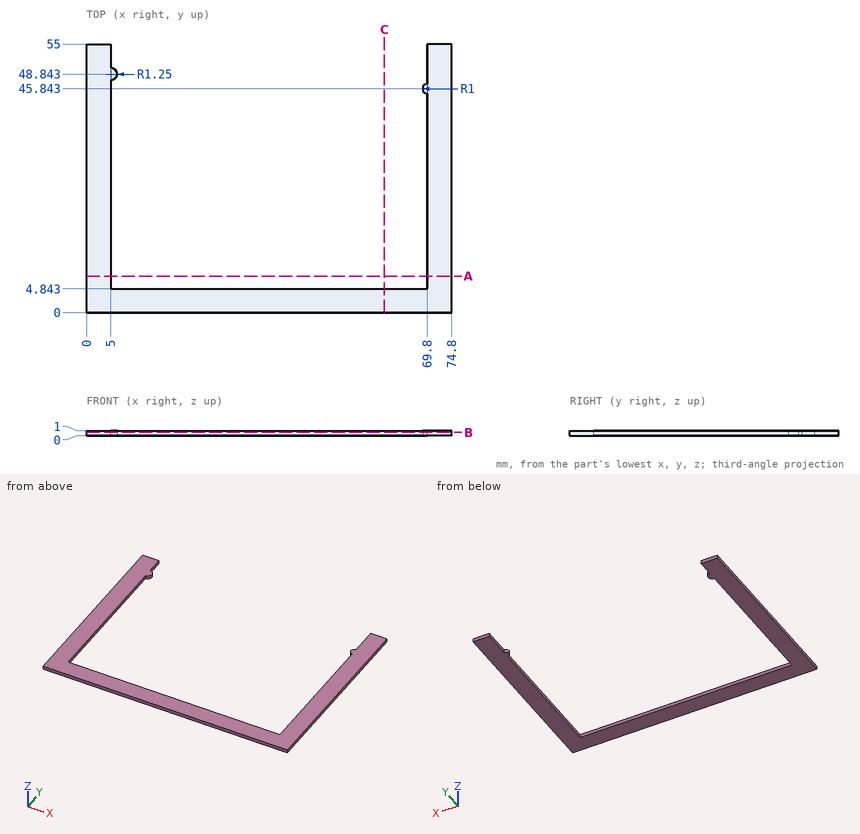
Here's the drawing with two shaded views (mm, measured from the low corner). I have some questions. Coordinates: 2 decimals unless noted, no trailing zeros. Write each loop counter-clockwise with the first axis right and the second up, starting at its lowest first coordinate (ties: lowest second). Pieces come first, ordered by that corner, then holes.
Item 1: I want a section at B-B on z = 0.65. Write out the boundary of the cut face in (x, y), and give its area (3 significant figures).
Item 2: If I drill on line 1 (X direction, y = 41, z = 0.75); line 2 (Y direction, x = 12, z = 0.35); line 3 (Y direction, x = 5.5, z = 0.4), over which ranges is the centre line in solid material (lowest first)?
Item 3: I want a section at A-A on y = 7.5. Write out the boundary of the cut face in (x, z), and give its area (3 significant figures).
Item 4: I want a section at C-C on x = 61. Write out the boundary of the cut face in (y, z).
Findings below:
1. outline: (0, 0) - (74.8, 0) - (74.8, 55) - (69.8, 55) - (69.8, 46.84) arc R1 ccw to (69.8, 44.84) - (69.8, 4.84) - (5, 4.84) - (5, 47.59) arc R1.25 ccw to (5, 50.09) - (5, 55) - (0, 55) - close
1. area: 868 mm2
2. line 1: x = 0 to 5, 69.8 to 74.8
2. line 2: y = 0 to 4.84
2. line 3: y = 0 to 4.84, 47.7 to 49.99
3. outline: (0, 0) - (5, 0) - (5, 1) - (0, 1) - close; (69.8, 0) - (74.8, 0) - (74.8, 1) - (69.8, 1) - close
3. area: 10.0 mm2
4. outline: (0, 0) - (4.84, 0) - (4.84, 1) - (0, 1) - close
